from build123d import *
from build123d.topology import SkipClean

# Parameters (mm, degrees)
SKETCH_2_R               = 7.5
EXTRUDE_1_DEPTH          = 10
EXTRUDE_START            = -40
SKETCH_2_3_R             = 7.5
EXTRUDE_2_DEPTH          = 10
SKETCH_3_R               = 7.5
SKETCH_3_R_2             = 5
SKETCH_3_R_3             = 11
EXTRUDE_3_DEPTH          = 50
CUT_EXTRUDE_2_DEPTH      = 121.623380818
CUT_EXTRUDE_2_DEPTH_BACK = 121.623380818
SKETCH_6_R               = 5
SKETCH_6_R_2             = 11


with BuildPart() as part:
    # Sketch 1 → Revolve 1 (revolve)
    with BuildSketch(Plane.XY, mode=Mode.PRIVATE) as revolve_1_sk:
        with BuildLine():
            Line((0, -11), (0, -35))
            Line((0, -35), (10, -35))
            Line((10, -35), (10, -15))
            Line((10, -15), (40, -15))
            Line((40, -15), (40, -35))
            Line((40, -35), (50, -35))
            Line((50, -35), (50, -20))
            Line((50, -20), (80, -20))
            Line((80, -20), (80, -25))
            Line((80, -25), (100, -25))
            ThreePointArc((100, -25), (107.071067812, -22.071067812), (110, -15))
            Line((110, -15), (110, -11))
            Line((110, -11), (0, -11))
        make_face()
    revolve(revolve_1_sk.sketch.rotate(Axis((0, 0, 0), (1, 0, 0)), 270), axis=Axis((0, 0, 0), (1, 0, 0)))

    # Sketch 2 → Extrude 1 (add)
    with BuildSketch(Plane.ZY):
        with BuildLine():
            Line((-25, 35), (25, 35))
            ThreePointArc((25, 35), (32.071067812, 32.071067812), (35, 25))
            Line((35, 25), (35, -25))
            ThreePointArc((35, -25), (32.071067812, -32.071067812), (25, -35))
            Line((25, -35), (-25, -35))
            ThreePointArc((-25, -35), (-32.071067812, -32.071067812), (-35, -25))
            Line((-35, -25), (-35, 25))
            ThreePointArc((-35, 25), (-32.071067812, 32.071067812), (-25, 35))
        make_face()
        with Locations((25, 25)):
            Circle(SKETCH_2_R, mode=Mode.SUBTRACT)
        with Locations((-25, 25)):
            Circle(SKETCH_2_R, mode=Mode.SUBTRACT)
        with Locations((-25, -25)):
            Circle(SKETCH_2_R, mode=Mode.SUBTRACT)
        with Locations((25, -25)):
            Circle(SKETCH_2_R, mode=Mode.SUBTRACT)
    extrude(amount=-EXTRUDE_1_DEPTH)

    # Sketch 2_3 → Extrude 2 (add)
    with BuildSketch(Plane.ZY.offset(EXTRUDE_START)):
        with BuildLine():
            Line((-25, 35), (25, 35))
            ThreePointArc((25, 35), (32.071067812, 32.071067812), (35, 25))
            Line((35, 25), (35, -25))
            ThreePointArc((35, -25), (32.071067812, -32.071067812), (25, -35))
            Line((25, -35), (-25, -35))
            ThreePointArc((-25, -35), (-32.071067812, -32.071067812), (-35, -25))
            Line((-35, -25), (-35, 25))
            ThreePointArc((-35, 25), (-32.071067812, 32.071067812), (-25, 35))
        make_face()
        with Locations((25, 25)):
            Circle(SKETCH_2_3_R, mode=Mode.SUBTRACT)
        with Locations((-25, 25)):
            Circle(SKETCH_2_3_R, mode=Mode.SUBTRACT)
        with Locations((-25, -25)):
            Circle(SKETCH_2_3_R, mode=Mode.SUBTRACT)
        with Locations((25, -25)):
            Circle(SKETCH_2_3_R, mode=Mode.SUBTRACT)
    extrude(amount=-EXTRUDE_2_DEPTH)

    # Sketch 3 → Extrude 3 (add)
    # profile 1 of 5: a face of its own
    with BuildSketch(Plane.ZY):
        with Locations((-25, 25)):
            Circle(SKETCH_3_R)
        with Locations(Location((-25, 25, 0), (0, 0, 36.869897646))):
            Circle(SKETCH_3_R_2, mode=Mode.SUBTRACT)
    # profile 2 of 5: a face of its own
    with BuildSketch(Plane.ZY):
        with Locations((25, 25)):
            Circle(SKETCH_3_R)
        with Locations(Location((25, 25, 0), (0, 0, 306.869897646))):
            Circle(SKETCH_3_R_2, mode=Mode.SUBTRACT)
    # profile 3 of 5: a face of its own
    with BuildSketch(Plane.ZY):
        with Locations((-25, -25)):
            Circle(SKETCH_3_R)
        with Locations(Location((-25, -25, 0), (0, 0, 323.130102354))):
            Circle(SKETCH_3_R_2, mode=Mode.SUBTRACT)
    # profile 4 of 5: a face of its own
    with BuildSketch(Plane.ZY):
        with Locations((25, -25)):
            Circle(SKETCH_3_R)
        with Locations(Location((25, -25, 0), (0, 0, 53.130102354))):
            Circle(SKETCH_3_R_2, mode=Mode.SUBTRACT)
    # profile 5 of 5: a face of its own
    with BuildSketch(Plane.ZY):
        Circle(SKETCH_3_R_3)
    extrude(amount=-EXTRUDE_3_DEPTH)

    # Sketch 6 → Cut-Extrude 2 (cut, two sides: drawn at the far end of the back side and taken through both)
    with SkipClean():  # the faces are left unmerged after this step: merging them gives an invalid solid
        with BuildSketch(Plane.ZY.offset(-CUT_EXTRUDE_2_DEPTH_BACK)):
            with Locations((-25, 25)):
                Circle(SKETCH_6_R)
            with Locations((-25, -25)):
                Circle(SKETCH_6_R)
            with Locations((25, 25)):
                Circle(SKETCH_6_R)
            with Locations((25, -25)):
                Circle(SKETCH_6_R)
            Circle(SKETCH_6_R_2)
        extrude(amount=CUT_EXTRUDE_2_DEPTH + CUT_EXTRUDE_2_DEPTH_BACK, mode=Mode.SUBTRACT)
    add(part.part.scale(1), mode=Mode.REPLACE)  # the faces are merged on a copy


solid = part.part
Here's how the part is built. I have some questions about the finished solid (model axes, mm). A direction names the side the tool comes from. Give positions to 0.01 mm unless a question says otherwise; leave off trailing zeros. Order: outer loops, then holes, each group sorted by start corner. A loop starts at its lowest first (then second) coordinate and runs counter-clockwise, first axis right, second up. Notation, with made-up numbers: M -10,55.5 L 44,55.5 A25 cw 44,74.5 Z; hole C 24,-10.5 d6. An arc over 180 degrees is marked long. Answer as a JSON object with one key per item and string values. Group by question number.
1) I'm going to push flat-ended pins straight in: pin 1 Ø2 at (x, y) = (38, 6.5) entering from +Z; pin 2 Ø1 at (y, z) = (2, 21.5) entering from +X; pin 3 Ø3 at (x, y) = (27.5, 1.5) entering from -Z; pin 4 Ø6 at (y, z) = (25, -25) entering from +X. Where does each tip first touch, or does it pass through?
2) Please list where these lines run through material, in increasing order: L1, parallel to Y at x = 15, z = 25; L2, parallel to Y at x = 19, z = 0; L3, parallel to X at y = 4, z = -15. Write a range as [from, to].
3) Suppose I cut it at D-D, the plane x = 82. Write out the boundary of the cut face in (y, z), plus the area to 3 significant figures.
4) Suppose I cut it at A-A, the plane y = 0. Write out the boundary of the cut face in (x, z).
5) We'd pull the mould along Z, two halves only. Please class faces 3 (the cylindrical face through (25.21, -0.66, -14.985)), 4 (the cylindrical face through (44.93, 31.99, -32.15)), 5 (the flat face through (40, 16, 0)): pulls with the +Z half, pulls with the -Z half, needs draft (parallel to the pull), parting line crosses it, or undercut.
6) Suppose I cut it at B-B, the plane z = -26.5. Write out the boundary of the cut face in (x, y).
7) On a 3-axis mill with a long thin cutter (end or side, diameter ignored), from which of +Z, -Z, +X, -X, +Y, -Y can I reach the whole of each face in a straight line? I mean faces 1 (the cylindrical face through (44.93, 32.15, 31.99)), 2 (the cylindrical face through (24.79, 22.13, 31.93)). Say none if no direction works.
Results found:
{
 "1": {"pin 1": "z = 13.96", "pin 2": "x = 107.93", "pin 3": "z = -15", "pin 4": "through"},
 "2": {"L1": "[-32.5, -30], [-20, -17.5], [17.5, 20], [30, 32.5]", "L2": "[-15, -11], [11, 15]", "L3": "[0, 10], [40, 109.99]"},
 "3": {"outline": "C 0,0 d50; hole C 0,0 d22", "area": "1,580 mm²"},
 "4": {"outline": "M 0,-35 L 10,-35 L 10,-15 L 40,-15 L 40,-35 L 50,-35 L 50,-20 L 80,-20 L 80,-25 L 100,-25 A10 ccw 110,-15 L 110,-11 L 0,-11 Z; M 0,11 L 110,11 L 110,15 A10 ccw 100,25 L 80,25 L 80,20 L 50,20 L 50,35 L 40,35 L 40,15 L 10,15 L 10,35 L 0,35 Z"},
 "5": {"face 3": "parting line crosses it", "face 4": "pulls with the -Z half", "face 5": "undercut"},
 "6": {"outline": "M 0,-34.89 L 10,-34.89 L 10,-32.35 L 40,-32.35 L 40,-34.89 L 50,-34.89 L 50,-29.77 L 0,-29.77 Z; M 0,-20.23 L 50,-20.23 L 50,20.23 L 0,20.23 Z; M 0,29.77 L 50,29.77 L 50,34.89 L 40,34.89 L 40,32.35 L 10,32.35 L 10,34.89 L 0,34.89 Z; hole M 10,-17.65 L 40,-17.65 L 40,17.65 L 10,17.65 Z"},
 "7": {"face 1": "+Z, +X, -X, +Y", "face 2": "none"}
}
